Here's how the part is built. I have some questions about the finished solid (model axes, mm). A direction names the side the tool comes from. Round coordinates to 2 decimals unless told otherwise and drop trailing zeros. Order: outer loops, then holes, each group sorted by start corner. A loop starts at its lowest first (then second) coordinate and runs counter-clockwise, first axis right, second up.
```python
from build123d import *

# Parameters (mm, degrees)
F1_DEPTH = 0.8
F2_DEPTH = 2


with BuildPart() as f1:
    # F0 (on Front) → F1 (new body)
    with BuildSketch(Plane.XZ):
        Polygon((25, 0), (0, 0), (0, 15.7), (14.3351472552, 22.7054297943), (11.8484024629, 27.0431827077), (-17.0050778452, 10.5020741364), (-4.685329569, -10.9878769608), (0.8098351958, -20.5733668117), (29.663315504, -4.0322582404), (27.3517045431, 0), align=None)
    extrude(amount=F1_DEPTH)

    # F0 (on Front) → F2 (join)
    with BuildSketch(Plane.XZ):
        Polygon((25, 0), (0, 0), (0, 15.7), (14.3351472552, 22.7054297943), (11.8484024629, 27.0431827077), (-17.0050778452, 10.5020741364), (-4.685329569, -10.9878769608), (0.8098351958, -20.5733668117), (29.663315504, -4.0322582404), (27.3517045431, 0), align=None)
        Polygon((0, 15.7), (0, 0), (20.5860966838, 11.8015870761), (14.3351472552, 22.7054297943), align=None)
        Polygon((20.5860966838, 11.8015870761), (0, 0), (25, 0), align=None)
        Polygon((20.5860966838, 11.8015870761), (25, 0), (27.3517045431, 0), (27.1765707117, 0.305494673), align=None)
    extrude(amount=-F2_DEPTH)


solid = f1.part
```
1. On a 3-axis mill with a long thin cutter (end or side, diameter ignored), from which of +Z, -Z, +X, -X, +Y, -Y can I reach the whole of each face in a straight line? I mean faces 1 (the flat face through (6, 2, 4)), 2 (the flat face through (10, 0, 9)). Say none if no direction works.
Evaluation:
face 1: +Z, -Z, +X, -X, +Y
face 2: +X, -Y
2. I need wall thicknesses on probe 1 along Y at (x, z) = (18, 2.5); probe 2 along X at (y, z) = (0.2, -5.5); probe 3 along Z at (x, y) = (11.5, -0.2). Which ranges of each line are inside material? Lowest first, please.
Evaluation:
probe 1: y = 0 to 2
probe 2: x = -7.83 to 27.1
probe 3: z = -14.44 to 0, 21.32 to 26.84
3. If we section it at C-C, the plane z = 1: Write out the boundary of the cut face in (x, y), and give its area (3 significant figures).
Evaluation:
outline: (-11.56, -0.8) - (0, -0.8) - (0, 0) - (26.78, 0) - (26.78, 2) - (-11.56, 2) - close
area: 85.9 mm2
4. If we mould it in two halves opening along Z, with no side actions, what happens to faces 3 (the flat face through (15.03, 0.58, -12.42)), 4 (the flat face through (4.5, -0.8, -0.2)), 5 (the flat face through (7.067, -0.394, 19.154))? For each: released by +Z, released by -Z, zero draft, split by the parting line, or undercut.
Evaluation:
face 3: released by -Z
face 4: zero draft
face 5: undercut
5. I'm going to push flat-ended pins straight in: P1, Ø1.5, axis at y = 1, z = 11, coming from the +X side; P2, Ø0.9, axis at x = 16.5, y = -0.5, coming from the +Z side; P3, Ø4, axis at x = 14.5, z = 6, coming from the -Y side. Where does each tip first touch, or does it pass through?
Evaluation:
P1: stops at x = 21.48
P2: stops at z = 0
P3: stops at y = 0
6. If we section it at D-D, the plane x = 2.5: Write out the boundary of the cut face in (y, z), and give its area (3 significant figures).
Evaluation:
outline: (-0.8, -19.6) - (2, -19.6) - (2, 21.68) - (-0.8, 21.68) - (-0.8, 16.92) - (0, 16.92) - (0, 0) - (-0.8, 0) - close
area: 102 mm2
7. If we section it at B-B, the plane x = 9.5: Write out the boundary of the cut face in (y, z).
Evaluation:
outline: (-0.8, -15.59) - (2, -15.59) - (2, 25.7) - (-0.8, 25.7) - (-0.8, 20.34) - (0, 20.34) - (0, 0) - (-0.8, 0) - close
8. If we section it at A-A, the plane y = 1.15: Write out the boundary of the cut face in (x, z).
Evaluation:
outline: (-17.01, 10.5) - (0.81, -20.57) - (29.66, -4.03) - (11.85, 27.04) - close
